Check sheet for the modelled part. Datum: model origin and axes. Units: mm. Face numbers are marked on the shaded views. A direction names the side the tool comes from. Coordinates: 2 decimals unless noted, no trailing zeros. Write each loop counter-clockwise with the first axis right and the second up, starting at its lowest first coordinate (ties: lowest second). Pieces come first, ordered by that corner, then holes. Notation, with made-up numbers: (76.5, 55) - (123.5, 55) arc R4 cw to (123.5, 62) - close; hole circle Ø5 at (-34, 11). An arc over 180 degrees is marked (long way). Write each question's results on one line, items separated by ' | '.
from build123d import *

# Parameters (mm, degrees)
SKETCH_1_W      = 42
SKETCH_1_H      = 26
SKETCH_1_R      = 1.25
EXTRUDE_1_DEPTH = 2
SKETCH_2_R      = 4
SKETCH_2_R_2    = 1.25
SKETCH_2_R_3    = 2
EXTRUDE_2_DEPTH = 2
SKETCH_3_W      = 8
SKETCH_3_H      = 26
SKETCH_3_R      = 2
EXTRUDE_3_DEPTH = 2
FILLET_1_R      = 2


with BuildPart() as part:
    # 草图1 → 凸台-拉伸1 (new body)
    with BuildSketch(Plane(origin=(0, 0, 0), x_dir=(1, 0, 0), z_dir=(0, 1, 0))):
        Rectangle(SKETCH_1_W, SKETCH_1_H)
        with Locations((10.75, 0)):
            Circle(SKETCH_1_R, mode=Mode.SUBTRACT)
        with Locations((3.75, 0)):
            Circle(SKETCH_1_R, mode=Mode.SUBTRACT)
        with Locations((10.75, 7)):
            Circle(SKETCH_1_R, mode=Mode.SUBTRACT)
        with Locations((17.75, 0)):
            Circle(SKETCH_1_R, mode=Mode.SUBTRACT)
        with Locations((10.75, -7)):
            Circle(SKETCH_1_R, mode=Mode.SUBTRACT)
        with Locations((-10.75, -7)):
            Circle(SKETCH_1_R, mode=Mode.SUBTRACT)
        with Locations((-17.75, 0)):
            Circle(SKETCH_1_R, mode=Mode.SUBTRACT)
        with Locations((-10.75, 0)):
            Circle(SKETCH_1_R, mode=Mode.SUBTRACT)
        with Locations((-10.75, 7)):
            Circle(SKETCH_1_R, mode=Mode.SUBTRACT)
        with Locations((-3.75, 0)):
            Circle(SKETCH_1_R, mode=Mode.SUBTRACT)
    extrude(amount=EXTRUDE_1_DEPTH)

    # 草图2 → 凸台-拉伸2 (add)
    with BuildSketch(Plane.XY.offset(13)):
        Polygon((21, 0), (-21, 0), (-21, 8), (-29, 8), (-29, 32.5), (-21, 32.5), (-21, 27.5), (-19, 27.5), (-19, 37.5), (0, 37.5), (19, 37.5), (19, 27.5), (21, 27.5), (21, 32.5), (29, 32.5), (29, 8), (21, 8), align=None)
        with Locations((0, 12)):
            Circle(SKETCH_2_R, mode=Mode.SUBTRACT)
        with Locations((0, 19)):
            Circle(SKETCH_2_R_2, mode=Mode.SUBTRACT)
        with Locations((7, 12)):
            Circle(SKETCH_2_R_2, mode=Mode.SUBTRACT)
        with Locations((0, 5)):
            Circle(SKETCH_2_R_2, mode=Mode.SUBTRACT)
        with Locations((-7, 12)):
            Circle(SKETCH_2_R_2, mode=Mode.SUBTRACT)
        with Locations((12, 22)):
            Circle(SKETCH_2_R, mode=Mode.SUBTRACT)
        with Locations((12, 29)):
            Circle(SKETCH_2_R_2, mode=Mode.SUBTRACT)
        with Locations((19, 22)):
            Circle(SKETCH_2_R_2, mode=Mode.SUBTRACT)
        with Locations((12, 15)):
            Circle(SKETCH_2_R_2, mode=Mode.SUBTRACT)
        with Locations((5, 22)):
            Circle(SKETCH_2_R_2, mode=Mode.SUBTRACT)
        with Locations((-19, 22)):
            Circle(SKETCH_2_R_2, mode=Mode.SUBTRACT)
        with Locations((-12, 15)):
            Circle(SKETCH_2_R_2, mode=Mode.SUBTRACT)
        with Locations((-12, 22)):
            Circle(SKETCH_2_R, mode=Mode.SUBTRACT)
        with Locations((-5, 22)):
            Circle(SKETCH_2_R_2, mode=Mode.SUBTRACT)
        with Locations((-12, 29)):
            Circle(SKETCH_2_R_2, mode=Mode.SUBTRACT)
        with Locations((-25, 22)):
            Circle(SKETCH_2_R_3, mode=Mode.SUBTRACT)
        with Locations((-25, 12)):
            Circle(SKETCH_2_R_3, mode=Mode.SUBTRACT)
        with Locations((25, 12)):
            Circle(SKETCH_2_R_3, mode=Mode.SUBTRACT)
        with Locations((25, 22)):
            Circle(SKETCH_2_R_3, mode=Mode.SUBTRACT)
    extrude(amount=-EXTRUDE_2_DEPTH)

    # 草图3 → 凸台-拉伸3 (add)
    with BuildSketch(Plane(origin=(0, 32.5, 0), x_dir=(1, 0, 0), z_dir=(0, 1, 0))):
        with Locations((-25, 0)):
            Rectangle(SKETCH_3_W, SKETCH_3_H)
        with Locations((-25, 5)):
            Circle(SKETCH_3_R, mode=Mode.SUBTRACT)
        with Locations((-25, -5)):
            Circle(SKETCH_3_R, mode=Mode.SUBTRACT)
        with Locations((25, 0)):
            Rectangle(SKETCH_3_W, SKETCH_3_H)
        with Locations((25, -5)):
            Circle(SKETCH_3_R, mode=Mode.SUBTRACT)
        with Locations((25, 5)):
            Circle(SKETCH_3_R, mode=Mode.SUBTRACT)
    extrude(amount=-EXTRUDE_3_DEPTH)

    # 圆角1
    fillet_1_edges = [part.edges().sort_by_distance(p)[0] for p in [
        (-25, 30.5, 11),
        (-29, 31.5, -13),
        (-21, 31.5, -13),
        (25, 30.5, 11),
        (21, 31.5, -13),
        (29, 31.5, -13),
        (0, 0, 13),
        (-29, 8, 12),
        (-19, 37.5, 12),
        (19, 37.5, 12),
        (29, 8, 12),
        (0, 2, 11),
        (25, 32.5, 13),
        (-25, 32.5, 13),
        (-21, 1, -13),
        (21, 1, -13),
    ]]
    fillet(fillet_1_edges, radius=FILLET_1_R)


solid = part.part
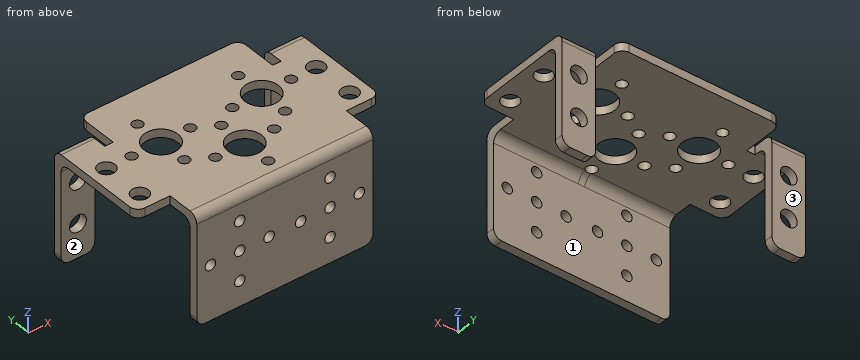
1. Sectioned sample at B-B (z = -10.25). Record the cut outline in (x, y).
Values follow:
outline: (-29, 30.5) - (-21, 30.5) - (-21, 32.5) - (-29, 32.5) - close; (-21, 0) - (21, 0) - (21, 2) - (-21, 2) - close; (21, 30.5) - (29, 30.5) - (29, 32.5) - (21, 32.5) - close
2. Go/stop test with flat-tipped pins: pin 1 (3 mm diameter, centred on x = -9.5, z = 7, fed in from +Y); pin 2 (10 mm diameter, centred on x = -12, y = 24.5, fed in from +Z); pin 3 (8 mm diameter, centred on x = -13.5, y = 30.5, fed in from -Z); pin 4 (2.5 mm diameter, centred on x = -24.5, z = 3, fed in from -Y). Record where each tip stops, or that it passes through.
Values follow:
pin 1: stops at y = 2 | pin 2: stops at z = 13 | pin 3: stops at z = 11 | pin 4: stops at y = 30.5
3. Sectioned sample at D-D (z = -5). Record the cut outline in (x, y).
Values follow:
outline: (-29, 30.5) - (-27, 30.5) - (-27, 32.5) - (-29, 32.5) - close; (-23, 30.5) - (-21, 30.5) - (-21, 32.5) - (-23, 32.5) - close; (-21, 0) - (21, 0) - (21, 2) - (-21, 2) - close; (21, 30.5) - (23, 30.5) - (23, 32.5) - (21, 32.5) - close; (27, 30.5) - (29, 30.5) - (29, 32.5) - (27, 32.5) - close
4. Sectioned sample at A-A (y = 12). Record the cut outline in (x, z), then the cut area to 3 significant figures.
Values follow:
outline: (-29, 11) - (-27, 11) - (-27, 13) - (-29, 13) - close; (-23, 11) - (-8.25, 11) - (-8.25, 13) - (-23, 13) - close; (-5.75, 11) - (-4, 11) - (-4, 13) - (-5.75, 13) - close; (4, 11) - (5.75, 11) - (5.75, 13) - (4, 13) - close; (8.25, 11) - (23, 11) - (23, 13) - (8.25, 13) - close; (27, 11) - (29, 11) - (29, 13) - (27, 13) - close | area: 74.0 mm^2
5. Sectioned sample at C-C (x = -7). Record the cut outline in (y, z), then the cut area to 3 significant figures.
Values follow:
outline: (0, -13) - (2, -13) - (2, 9) arc R2 cw to (4, 11) - (10.75, 11) - (10.75, 13) - (2, 13) arc R2 ccw to (0, 11) - close; (13.25, 11) - (37.5, 11) - (37.5, 13) - (13.25, 13) - close | area: 118 mm^2
6. Material ranges on L1, parallel to X at y = 31.9, z = 5; L2, parallel to Y at x = -12, z = 11.8; L3, parallel to Y at x = -26, z = 12, recorded low to high. Write a range as [from, to].
Values follow:
L1: x = [-29, -27], [-23, -21], [21, 23], [27, 29] | L2: y = [0.17, 13.75], [16.25, 18], [26, 27.75], [30.25, 37.5] | L3: y = [8, 10.27], [13.73, 20.27], [23.73, 32.23]
7. Access from +Z, -Z, +X, -X, +Y, -Y to the whole of each face (thin tool, end or side, straight path). Record for the marked faces 1, 2 and 3.
Values follow:
face 1: -Z, +X, -X, +Y | face 2: -Z, +X, -X, -Y | face 3: +Z, -Z, +X, -X, +Y
